For this review, take the finished solid that the model builds, in its own axes (mm). A direction names the side the tool comes from. Round coordinates to 2 decimals unless told otherwise and drop trailing zeros. Write each loop counter-clockwise with the first axis right and the second up, starting at its lowest first coordinate (ties: lowest second). Pieces come first, ordered by that corner, then holes. Notation, with made-up numbers: (39, 2) -> (75, 2) arc R20 ccw to (75, 36) -> close; hole circle Ø2 at (-30, -30.5). An arc over 180 degrees is marked (long way). Write item = value, one per line. Start each with the question number.
```python
from build123d import *

# Parameters (mm, degrees)
ESBO_O1_R                = 1.499999648
ESBO_O1_R_2              = 1.500000298
ESBO_O1_R_3              = 7.49999945
ESBO_O1_R_4              = 1.49999992
ESBO_O1_R_5              = 2.500000663
ESBO_O1_R_6              = 2.499999944
ESBO_O1_R_7              = 1.500000264
ESBO_O1_R_8              = 2.499997616
ESBO_O1_R_9              = 2.499998574
ESBO_O1_R_10             = 2.500000277
ESBO_O1_R_11             = 1.500000402
ESBO_O1_R_12             = 1.500002802
ESBO_O1_R_13             = 1.500001991
ESBO_O1_R_14             = 5.000001307
ESBO_O1_R_15             = 1.500000261
RESSALTO_EXTRUS_O1_DEPTH = 6


with BuildPart() as part:
    # Esboço1 → Ressalto-extrusão1 (new body)
    with BuildSketch(Plane.XY):
        Polygon((-39.385000246, 159.55550476), (0.115000002, 159.55550476), (0.115000002, -55.444498231), (-39.384998091, -55.444498231), (-64.385000326, -20.944499718), (-112.38500214, -20.944499718), (-114.885002049, -18.444498377), (-114.885002049, 122.555504246), (-112.385001967, 125.055501899), (-64.385002481, 125.055501899), align=None)
        with Locations((-110.885001778, 0.055499999)):
            Circle(ESBO_O1_R, mode=Mode.SUBTRACT)
        with Locations((-93.885001436, 0.055499999)):
            Circle(ESBO_O1_R_2, mode=Mode.SUBTRACT)
        with Locations((-102.385001898, -8.444500463)):
            Circle(ESBO_O1_R_3, mode=Mode.SUBTRACT)
        with Locations((-110.885002127, -16.944500925)):
            Circle(ESBO_O1_R_4, mode=Mode.SUBTRACT)
        with Locations((-29.885004915, -25.444498593)):
            Circle(ESBO_O1_R_5, mode=Mode.SUBTRACT)
        with Locations((-9.885005362, -45.444498612)):
            Circle(ESBO_O1_R_6, mode=Mode.SUBTRACT)
        with Locations((-93.885002367, -16.944499062)):
            Circle(ESBO_O1_R_7, mode=Mode.SUBTRACT)
        with Locations((-29.88500119, 52.055502934)):
            Circle(ESBO_O1_R_8, mode=Mode.SUBTRACT)
        with Locations((-9.885001637, 149.555499358)):
            Circle(ESBO_O1_R_9, mode=Mode.SUBTRACT)
        with Locations((-29.88500119, 129.55550353)):
            Circle(ESBO_O1_R_10, mode=Mode.SUBTRACT)
        with Locations((-102.385000966, 60.055504246)):
            Circle(ESBO_O1_R_11, mode=Mode.SUBTRACT)
        with Locations((-94.385001518, 52.055502934)):
            Circle(ESBO_O1_R_12, mode=Mode.SUBTRACT)
        with Locations((-110.385000997, 52.055502934)):
            Circle(ESBO_O1_R_13, mode=Mode.SUBTRACT)
        with Locations((-102.385000966, 52.055502934)):
            Circle(ESBO_O1_R_14, mode=Mode.SUBTRACT)
        with Locations((-102.385000966, 44.055505348)):
            Circle(ESBO_O1_R_15, mode=Mode.SUBTRACT)
        with Locations((-93.885002367, 121.055504931)):
            Circle(ESBO_O1_R_7, mode=Mode.SUBTRACT)
        with Locations((-110.885002127, 121.055506794)):
            Circle(ESBO_O1_R_4, mode=Mode.SUBTRACT)
        with Locations((-102.385001898, 112.555506332)):
            Circle(ESBO_O1_R_3, mode=Mode.SUBTRACT)
        with Locations((-93.885001436, 104.05550587)):
            Circle(ESBO_O1_R_2, mode=Mode.SUBTRACT)
        with Locations((-110.885001778, 104.05550587)):
            Circle(ESBO_O1_R, mode=Mode.SUBTRACT)
    extrude(amount=RESSALTO_EXTRUS_O1_DEPTH)


solid = part.part
```
1. Machinability: for faces 1 (the flat face through (0.115, 54, 3)), 2 (the flat face through (-88, -20.944, 3)), which of the approach directions +Z, -Z, +X, -X, +Y, -Y give a long, thin tool a straight path to every point of the face, cutting with its end or side? Answer none if there is none.
2. Draft analysis for pull direction X (two halves, no side actions). For faces 3 (the cylindrical face through (-27.5, -24.7, 3)), 4 (the flat face through (-89, 125.056, 3)), 5 (the flat face through (-52.06, 142.064, 2.958)), state which applies: +X half, -X half, draft (parallel to the pull), parting line (faces both ways), or undercut.
3. Consider section C-C, the plane x = -57.5. Give the boundary of the cut face in (y, z), then the cut area to 3 significant figures.
4. Wall thickness on L1, parallel to Y at x = -29, z = 2.75; L2, parallel to Y at x = -100, z = 4.15; L3, parallel to Y at x = -66.5, z = 5.35: over which ranges is each line inside the solid? List them lowest first. Write a range as from..to.
5. Clearance check with flat-ended pins moving along their axes: pin 1 Ø11.5 at (x, y) = (-102.39, 52.06) entering from -Z; pin 2 Ø3 at (x, y) = (-29.89, -25.44) entering from -Z; pin 3 Ø1.8 at (x, z) = (-85, 2) entering from +Y. State where each tip first meets the part, or that it passes through.
6. Consider section A-A, the plane z = 1.6. Give the number of separate pieces and of enclosed holes in the cut face, then the cut area to 3 significant figures.
7. Consider section B-B, the plane x = -89. Give the boundary of the cut face in (y, z), then the cut area to 3 significant figures.
Outcome:
q1.face_1 = +Z, -Z, +X, +Y, -Y
q1.face_2 = +Z, -Z, -X, -Y
q2.face_3 = undercut
q2.face_4 = draft
q2.face_5 = -X half
q3.outline = (-30.45, 0) -> (134.56, 0) -> (134.56, 6) -> (-30.45, 6) -> close
q3.area = 990 mm2
q4.L1 = -55.44..-27.78, -23.11..49.72, 54.39..127.22, 131.89..159.56
q4.L2 = -20.94..-15.56, -1.33..47.66, 56.45..105.44, 119.67..125.06
q4.L3 = -20.94..125.06
q5.pin_1 = 0
q5.pin_2 = through
q5.pin_3 = 125.06
q6.separate_pieces = 1
q6.enclosed_holes = 20
q6.area = 19,800 mm2
q7.outline = (-20.94, 0) -> (125.06, 0) -> (125.06, 6) -> (-20.94, 6) -> close
q7.area = 876 mm2
